Could you check a few things on this model? Use its own coordinates, in mm. Face numbers are marked on the shaded views. A direction names the side the tool comes from. Coordinates: 2 decimals unless noted, no trailing zeros. Order: outer loops, then holes, each group sorted by start corner. A loop starts at its lowest first (then second) coordinate and runs counter-clockwise, first axis right, second up. Notation, with made-up numbers: (4, -14.75) -> (20, -14.75) arc R17 ccw to (20, 18.25) -> close; hole circle Ø2 at (-38.5, -23). An arc over 180 degrees is marked (long way). Use a Markdown table: item, result. Add a question column.
1) If we section it at A-A (x = 0): Write out the boundary of the cut face in (y, z), plus the area to 3 significant figures.
2) If we section it at C-C (z = 0): Write out the boundary of the cut face in (x, y), plus the area to 3 significant figures.
3) If we section it at B-B (y = -5): Write out the boundary of the cut face in (x, z).
4) If we section it at D-D (y = 1.25): Write out the boundary of the cut face in (x, z), plus the area to 3 significant figures.
5) If I drill on L1, parallel to X at y = 0.7, z = 0; L2, parallel to Y at x = 2.75, z = 8.75; L3, parallel to Y at x = 0, z = 10.9, over which ranges is the centre line in solid material (lowest first)? Write a range as [from, to].
6) Thinking about a two-plate mould opening in Z: for the marked faces 3, 4 and 5, which applies, +Z half, -Z half, draft (parallel to the pull), parting line (faces both ways), or undercut?
7) Which directions (+Z, -Z, +X, -X, +Y, -Y) give clear straight access to the entire face, cutting with the end or side of a thin tool? Please do the marked faces 1 and 2.
8) Will these pins go through, and if not, where does the flat tip stop? pin 1 Ø3.5 at (x, z) = (0, 0) entering from -Y; pin 2 Ø2 at (x, y) = (1, -6.5) entering from -Z.
```python
from build123d import *

# Parameters (mm, degrees)
SKETCH1_W           = 10
SKETCH1_H           = 18
SKETCH1_R           = 1.5
BOSS_EXTRUDE1_DEPTH = 3
SKETCH2_W           = 10
SKETCH2_H           = 3
BOSS_EXTRUDE2_DEPTH = 10
SKETCH3_R           = 1.5
CUT_EXTRUDE1_DEPTH  = 22.1896201


with BuildPart() as part:
    # Sketch1 → Boss-Extrude1 (new body)
    with BuildSketch(Plane(origin=(0, 0, 0), x_dir=(1, 0, 0), z_dir=(0, 1, 0))):
        with Locations((0, -4)):
            Rectangle(SKETCH1_W, SKETCH1_H)
        with Locations(Location((0, 0, 0), (0, 0, 270))):
            Circle(SKETCH1_R, mode=Mode.SUBTRACT)
    extrude(amount=BOSS_EXTRUDE1_DEPTH)

    # Sketch2 → Boss-Extrude2 (add)
    with BuildSketch(Plane.XZ):
        with Locations((0, 11.5)):
            Rectangle(SKETCH2_W, SKETCH2_H)
    extrude(amount=BOSS_EXTRUDE2_DEPTH)

    # Sketch3 → Cut-Extrude1 (cut, through all)
    with BuildSketch(Plane.XY.offset(13)):
        with Locations((0, -5)):
            Circle(SKETCH3_R)
    extrude(amount=-CUT_EXTRUDE1_DEPTH, mode=Mode.SUBTRACT)


solid = part.part
```
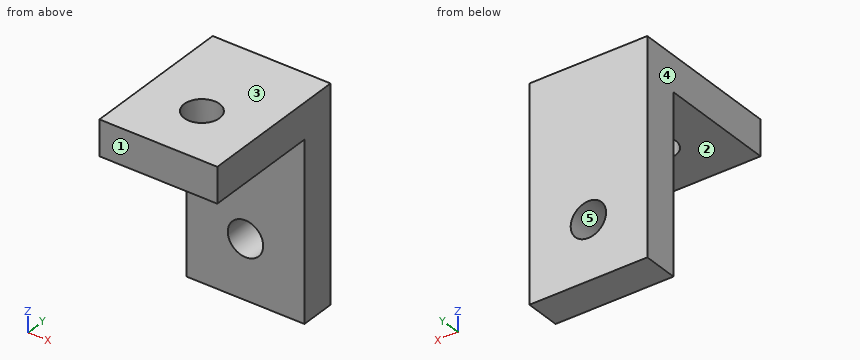
Answer sheet:
| question | item | result |
|---|---|---|
| 1 | outline | (-10, 10) -> (-6.5, 10) -> (-6.5, 13) -> (-10, 13) -> close; (-3.5, 10) -> (0, 10) -> (0, 1.5) -> (3, 1.5) -> (3, 13) -> (-3.5, 13) -> close; (0, -5) -> (3, -5) -> (3, -1.5) -> (0, -1.5) -> close |
| 1 | area | 66.0 mm2 |
| 2 | outline | (-5, 0) -> (-1.5, 0) -> (-1.5, 3) -> (-5, 3) -> close; (1.5, 0) -> (5, 0) -> (5, 3) -> (1.5, 3) -> close |
| 2 | area | 21.0 mm2 |
| 3 | outline | (-5, 10) -> (-1.5, 10) -> (-1.5, 13) -> (-5, 13) -> close; (1.5, 10) -> (5, 10) -> (5, 13) -> (1.5, 13) -> close |
| 4 | outline | (-5, -5) -> (5, -5) -> (5, 13) -> (-5, 13) -> close; hole circle Ø3 at (0, 0) |
| 4 | area | 173 mm2 |
| 5 | L1 | [-5, -1.5], [1.5, 5] |
| 5 | L2 | [0, 3] |
| 5 | L3 | [-10, -6.5], [-3.5, 3] |
| 6 | face 3 | +Z half |
| 6 | face 4 | draft |
| 6 | face 5 | undercut |
| 7 | face 1 | +Z, -Z, +X, -X, -Y |
| 7 | face 2 | -Z, +X, -X, -Y |
| 8 | pin 1 | y = 0 |
| 8 | pin 2 | z = 10 |
